Autodesk Inventor part; units mm, degrees
ref_plane "YZ Plane" through (0, 0, 0) normal (1, 0, 0) x (0, 1, 0)
ref_plane "XZ Plane" through (0, 0, 0) normal (0, 1, 0) x (-1, 0, 0)
ref_plane "XY Plane" through (0, 0, 0) normal (0, 0, 1) x (1, 0, 0)
sketch "Skizze1" plane through (0, 0, 0) normal (0, 0, 1) x (1, 0, 0)
  line L0 (0, 0) -> (7.85, 0)
  line L1 (3.925, 0) -> (3.925, 15.4029) construction
  line L2 (0, 0) -> (0, 6)
  line L3 (0, 6) -> (2, 6)
  line L4 (2, 6) -> (3.425, 4.575)
  line L5 (3.425, 4.575) -> (3.425, 4.5)
  arc A0 (3.425, 4.5) -> (4.425, 4.5) centre (3.925, 4.5) ccw
  line L6 (4.425, 4.5) -> (4.425, 4.575)
  line L7 (4.425, 4.575) -> (5.85, 6)
  line L8 (5.85, 6) -> (7.85, 6)
  line L9 (7.85, 6) -> (7.85, 0)
  dimension "d0" = 2
  dimension "d1" = 45
  dimension "d2" = 0.5
  dimension "d3" = 12
  dimension "d4" = 9
  dimension "d5" = 7.85
revolve "Umdrehung1" add sketch "Skizze1" angle 360 about axis through (0, 0, 0) along (1, 0, 0)
sketch "Skizze2" plane through (7.85, 0, 0) normal (1, 0, 0) x (0, 0, -1)
  circle A0 centre (0, 0) radius 6
  circle A1 centre (0, 0) radius 1.5
  line L0 (-0.869, 1.2226) -> (-2.469, 2.8225)
  line L1 (-1.2226, 0.869) -> (-2.8225, 2.469)
  line L2 (8.4, 0) -> (-8.4, 0)
  line L3 (0, 0) -> (-2.6517, 2.6517) construction
  circle A2 centre (0, 0) radius 3.75
  line L4 (-1.5, 0) -> (-3.75, 0)
  dimension "d7" = 3
  dimension "d8" = 45
  dimension "d9" = 0.5
  dimension "d10" = 7.5
extrude "Extrusion2" cut sketch "Skizze2" against normal through all contours A2 L1 A1 L2
pattern_circular "Runde Anordnung2" count 6 over 360 about axis through (6.85, 0, 0) along (1, 0, 0) of "Extrusion2"
sketch "Skizze3" plane through (7.85, 0, 0) normal (1, 0, 0) x (0, 0, -1)
  circle A0 centre (0, 0) radius 0.9
  dimension "d21" = 1.8
extrude "Extrusion3" cut sketch "Skizze3" against normal up to surface (7.85 mm away)
properties part number "Rad" material "Stahl, galvanisiert"
Design review of the part built by this model. Coordinates are the model's own, in mm. Coordinates: 2 decimals unless noted, no trailing zeros.
1) Wall thickness on line 1 along Y through (x, z) = (5.5, 0); line 2 along Z through (x, y) = (4.25, 1.75); line 3 along Z through (x, y) = (3, 0.5): over which ranges is each line inside the solid? List them lowest first.
2) Clearance check with flat-ended pins moving along their axes: pin 1 (1 mm diameter, centred on x = 2.5, y = -2.5, fed in from +Z); pin 2 (1 mm diameter, centred on x = 3, z = 0.5, fed in from -Y); pin 3 (1.5 mm diameter, centred on x = 4, z = 2, fed in from -Y); pin 4 (1.1 mm diameter, centred on y = 0, z = 0, fed in from -X). State where each tip first meets the part, or that it passes through.
3) Mouldability with a two-part tool opening along Y and no side actions: class faces 1 (the flat face through (4, 0, -3)), 2 (the flat face through (3.98, -1.658, -2.011)), 3 (the flat face through (7.85, 1.2, 0.1)) as +Y half, -Y half, draft (parallel to the pull), parting line (faces both ways), or undercut.
4) Take a section at A-A, the plane x = 1. State how many separate pieces and enclosed holes the cut face has, and give its area (3 significant figures).
Returned:
1. line 1: y = -5.65 to -3.75, -1.5 to -0.9, 0.9 to 1.5, 3.75 to 5.65
1. line 2: z = -3.73 to -3.32, -1.01 to -0.21, 1.01 to 2.1, 3.32 to 3.73
1. line 3: z = -4.97 to -0.75, 0.75 to 1.41, 3.72 to 4.97
2. pin 1: stops at z = 5.5
2. pin 2: stops at y = -5.48
2. pin 3: stops at y = -4.53
2. pin 4: passes through
3. face 1: undercut
3. face 2: undercut
3. face 3: draft
4. separate pieces: 1
4. enclosed holes: 7
4. area: 86.1 mm2
